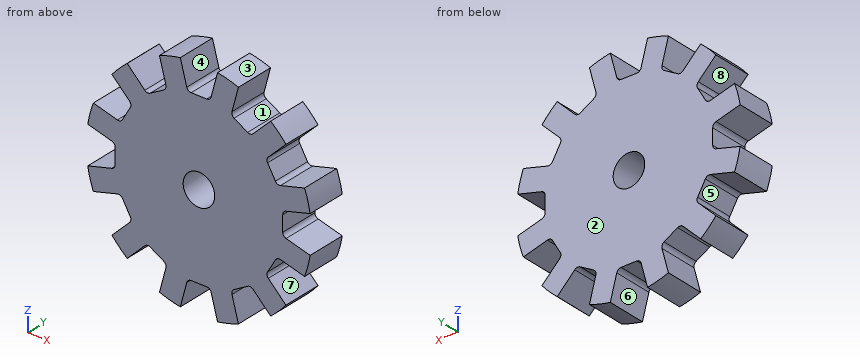
from build123d import *

# Parameters (mm, degrees)
F0_R     = 25.4
F1_DEPTH = 8.89
F3_DEPTH = 25.4
F4_COUNT = 12
F4_ANGLE = 330
F5_R     = 3.556
F6_DEPTH = 25.4


with BuildPart() as f1:
    # F0 (on Front) → F1 (new body)
    with BuildSketch(Plane.XZ):
        Circle(F0_R)
    extrude(amount=F1_DEPTH)

    # F2 (on face) → F3 (cut)
    with BuildSketch(Plane.XZ.offset(8.89)):
        with BuildLine():
            ThreePointArc((1.7603957802, 18.8799073091), (2.3788973921, 19.0898603154), (2.7417764197, 19.6329471593))
            Line((2.7417764197, 19.6329471593), (4.19365, 25.0514131273))
            ThreePointArc((4.19365, 25.0514131274), (0, 25.4), (-4.19365, 25.0514131274))
            Line((-4.19365, 25.0514131273), (-2.7417764197, 19.6329471593))
            ThreePointArc((-2.7417764197, 19.6329471593), (-2.3788973921, 19.0898603154), (-1.7603957802, 18.8799073091))
            Line((-1.7603957802, 18.8799073091), (0, 18.8799073091))
            Line((0, 18.8799073091), (1.7603957802, 18.8799073091))
        make_face()
    f3 = extrude(amount=-F3_DEPTH, mode=Mode.SUBTRACT)

    # F4: F3 ×12 about axis
    f4_axis = Axis((0, 0, 0), (0, 1, 0))
    for i in range(1, F4_COUNT):
        add(f3.rotate(f4_axis, i * F4_ANGLE / (F4_COUNT - 1)), mode=Mode.SUBTRACT)

    # F5 (on face) → F6 (cut)
    with BuildSketch(Plane.XZ.offset(8.89)):
        Circle(F5_R)
    extrude(amount=-F6_DEPTH, mode=Mode.SUBTRACT)


solid = f1.part
Verification items for the finished model (mm, model axes). Face numbers are marked on the shaded views. A direction names the side the tool comes from. Give positions to 0.01 mm unless a question says otherwise; leave off trailing zeros. Order: outer loops, then holes, each group sorted by start corner. A loop starts at its lowest first (then second) coordinate and runs counter-clockwise, first axis right, second up. Notation, with made-up numbers: (80, 26.5) -> (97, 26.5) arc R18 cw to (97, 33.5) -> close; hole circle Ø8 at (-2, 7). An arc over 180 degrees is marked (long way). Answer as CSV lines item,"result".
Q1. Sectioned sample at A-A on z = 0. Record the cut outline in (x, y), plus the area to 3 significant figures.
Solutions:
outline,"(-18.88, -8.89) -> (-3.56, -8.89) -> (-3.56, 0) -> (-18.88, 0) -> close; (3.56, -8.89) -> (18.88, -8.89) -> (18.88, 0) -> (3.56, 0) -> close"
area,"272 mm²"
Q2. Scan lines: probe 1 along X at (y, z) = (-6, -17); probe 2 along Z at (x, y) = (0, -2.5); probe 3 along Z at (x, y) = (-19.5, -2.75). Record each from-to range of solid material in increasing order.
Solutions:
probe 1,"x = -18.87 to -13.56, -8.31 to 8.31, 13.56 to 18.87"
probe 2,"z = -18.88 to -3.56, 3.56 to 18.88"
probe 3,"z = -16.28 to -16.06, -7.74 to -2.7, 2.7 to 7.74, 16.06 to 16.28"
Q3. Access from +Z, -Z, +X, -X, +Y, -Y to the whole of each face (thin tool, end or side, straight path). Record for the marked faces 4, 5, 6, 7 and 8.
Solutions:
face 4,"+Z, +Y, -Y"
face 5,"+Y, -Y"
face 6,"-Z, +Y, -Y"
face 7,"+X, +Y, -Y"
face 8,"-X, +Y, -Y"
Q4. Sectioned sample at B-B on x = 0. Record the cut outline in (y, z), plus the area to 3 significant figures.
Solutions:
outline,"(-8.89, -18.88) -> (0, -18.88) -> (0, -3.56) -> (-8.89, -3.56) -> close; (-8.89, 3.56) -> (0, 3.56) -> (0, 18.88) -> (-8.89, 18.88) -> close"
area,"272 mm²"
Q5. Sectioned sample at C-C on z = 10. Record the cut outline in (x, y), plus the area to 3 significant figures.
Solutions:
outline,"(-16.03, -8.89) -> (16.03, -8.89) -> (16.03, 0) -> (-16.03, 0) -> close"
area,"285 mm²"
Q6. Depth check by flat-ended pin: pin 1 (3 mm diameter, centred on x = -10.5, y = -5.5, fed in from -Z); pin 2 (1.1 mm diameter, centred on x = -0.5, y = -5, fed in from +Z); pin 3 (3 mm diameter, centred on x = -13.5, y = -2.5, fed in from +Z). Enter the tip coordinate at first touch or a pass-through.
Solutions:
pin 1,"stops at z = -16.6"
pin 2,"stops at z = 18.88"
pin 3,"stops at z = 18.44"
Q7. Sectioned sample at D-D on x = 10. Record the cut outline in (y, z), plus the area to 3 significant figures.
Solutions:
outline,"(-8.89, -16.03) -> (0, -16.03) -> (0, 16.03) -> (-8.89, 16.03) -> close"
area,"285 mm²"
Q8. Release check for a two-part mould opening along Z. For the marked faces 1, 2 and 3 record: +Z half, -Z half, draft (parallel to the pull), parting line (faces both ways), or undercut.
Solutions:
face 1,"undercut"
face 2,"draft"
face 3,"+Z half"
